from build123d import *

# Parameters (mm, degrees)
BOSS_EXTRUDE1_DEPTH = 5
BOSS_EXTRUDE2_DEPTH = 20
SKETCH4_W           = 55
SKETCH4_H           = 4
BOSS_EXTRUDE3_DEPTH = 20
SKETCH6_R           = 1.8
CUT_EXTRUDE3_DEPTH  = 6


with BuildPart() as part:
    # Sketch1 → Boss-Extrude1 (new body)
    with BuildSketch(Plane.XY):
        Polygon((14.31372549, -4.264705882), (34.31372549, -4.264705882), (34.31372549, -19.264705882), (-20.68627451, -19.264705882), (-20.68627451, -4.264705882), (-0.68627451, -4.264705882), (-0.68627451, 15.735294118), (14.31372549, 15.735294118), align=None)
    extrude(amount=BOSS_EXTRUDE1_DEPTH)

    # Sketch2 → Boss-Extrude2 (add)
    with BuildSketch(Plane(origin=(0, 0, 0), x_dir=(-1, 0, 0), z_dir=(0, 0, -1))):
        Polygon((0.68627451, 15.735294118), (4.68627451, 15.735294118), (4.68627451, -0.264705882), (6.079970528, -0.264705882), (20.68627451, -0.264705882), (20.68627451, -4.264705882), (0.68627451, -4.264705882), align=None)
    boss_extrude2 = extrude(amount=-BOSS_EXTRUDE2_DEPTH)

    # Sketch4 → Boss-Extrude3 (add)
    with BuildSketch(Plane(origin=(0, 0, 0), x_dir=(-1, 0, 0), z_dir=(0, 0, -1))):
        with Locations((-6.81372549, -21.264705882)):
            Rectangle(SKETCH4_W, SKETCH4_H)
    extrude(amount=-BOSS_EXTRUDE3_DEPTH)

    # Mirror1: Boss-Extrude2 across plane
    add(boss_extrude2.mirror(Plane.ZY.offset(-6.81372549)))

    # Sketch6 → Cut-Extrude3 (cut, through all)
    with BuildSketch(Plane.XY.offset(5)):
        with Locations((6.81372549, 8.235294118)):
            Circle(SKETCH6_R)
        with Locations((-13.18627451, -11.764705882)):
            Circle(SKETCH6_R)
        with Locations((26.81372549, -11.764705882)):
            Circle(SKETCH6_R)
    extrude(amount=-CUT_EXTRUDE3_DEPTH, mode=Mode.SUBTRACT)


solid = part.part
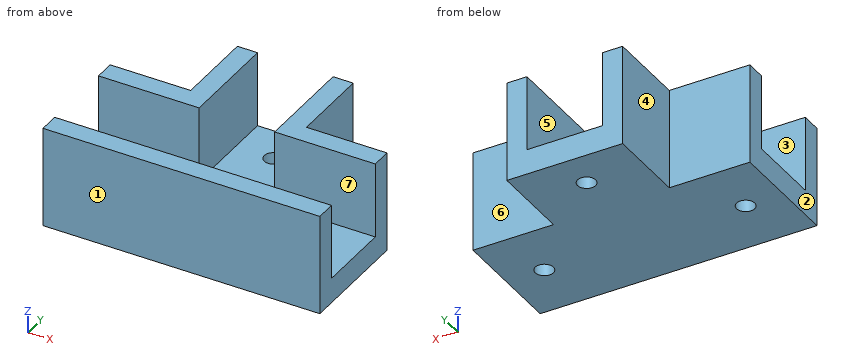
Read the model definition and answer for the solid it produces. Units are mm, in the model's axes. Face numbers are marked on the shaded views. A direction names the side the tool comes from. Coordinates: 2 decimals unless noted, no trailing zeros. Loops run counter-clockwise (first coordinate to the right, second up) from the corner with the lowest first, then second, coordinate; pieces in that order, holes last.
Q1. The part is cut by section A-A on z = 9.5. Write down the section's boundary in (x, y).
Q2. The mould has two halves that part along Y. Classify the marked faces 1, 2 and 3: +Y half, -Y half, draft (parallel to the pull), parting line (faces both ways), or undercut.
Q3. The part is cut by section B-B on x = 26. Write down the section's boundary in (y, z), and give its area (3 significant figures).
Q4. Each of these flat-tipped pins is pushed along its axis until it touches: pin 1 Ø8 at (x, z) = (-9, 10.5) entering from +Y; pin 2 Ø2 at (x, y) = (6.81, 8.24) entering from -Z; pin 3 Ø10.5 at (x, y) = (1, 1.5) entering from +Z; pin 4 Ø12 at (y, z) = (10, 14) entering from +X. Where does it stop, or does it pass through?
Q5. The part is cut by section C-C on y = -2. Write down the section's boundary in (x, z), and give its area (3 significant figures).
Q6. The part is cut by section D-D on x = -17. Write down the section's boundary in (y, z).
Q7. Which of the six approach directions +Z, -Z, +X, -X, +Y, -Y give full straight-line access (tool end or side, diameter ignored) to the marked faces 4, 5, 6 and 7?
Q8. Consider probe 1 along Y at (x, z) = (31, 19); probe 2 along X at (y, z) = (2.5, 6.5); probe 3 along X at (y, z) = (-1.5, 10.5). Determine where each line is inside the solid, lowest interval first.
Results below:
1. outline: (-20.69, -23.26) - (34.31, -23.26) - (34.31, -19.26) - (-20.69, -19.26) - close; (-20.69, -4.26) - (-0.69, -4.26) - (-0.69, 15.74) - (-4.69, 15.74) - (-4.69, -0.26) - (-20.69, -0.26) - close; (14.31, -4.26) - (34.31, -4.26) - (34.31, -0.26) - (18.31, -0.26) - (18.31, 15.74) - (14.31, 15.74) - close
2. face 1: -Y half
2. face 2: draft
2. face 3: undercut
3. outline: (-23.26, 0) - (-13.37, 0) - (-13.37, 5) - (-19.26, 5) - (-19.26, 20) - (-23.26, 20) - close; (-10.16, 0) - (-0.26, 0) - (-0.26, 20) - (-4.26, 20) - (-4.26, 5) - (-10.16, 5) - close
3. area: 219 mm2
4. pin 1: stops at y = -0.26
4. pin 2: passes through
4. pin 3: stops at z = 20
4. pin 4: stops at x = 18.31
5. outline: (-20.69, 0) - (34.31, 0) - (34.31, 20) - (14.31, 20) - (14.31, 5) - (-0.69, 5) - (-0.69, 20) - (-20.69, 20) - close
5. area: 875 mm2
6. outline: (-23.26, 0) - (-0.26, 0) - (-0.26, 20) - (-4.26, 20) - (-4.26, 5) - (-19.26, 5) - (-19.26, 20) - (-23.26, 20) - close
7. face 4: +Z, -Z, -X, +Y
7. face 5: +Z, +Y
7. face 6: +Z, -Z, +X, +Y
7. face 7: +Z, +X, -X
8. probe 1: y = -23.26 to -19.26, -4.26 to -0.26
8. probe 2: x = -4.69 to -0.69, 14.31 to 18.31
8. probe 3: x = -20.69 to -0.69, 14.31 to 34.31
